Part model, mm, in its own coordinate system. Round coordinates to 2 decimals unless told otherwise and drop trailing zeros. Write each loop counter-clockwise with the first axis right and the second up, starting at its lowest first coordinate (ties: lowest second). Pieces come first, ordered by that corner, then holes. Notation, with made-up numbers: M -24.5,69 L 22.5,69 A30 ccw 22.5,105 Z; hole C 11.5,-20 d7. An arc over 180 degrees is marked long. Use a Markdown table: item, result. Add a question column.
1) Slice it at B-B on z = 0. Write the cut outline in (x, y), plus the area to 4 significant figures.
2) Slice it at D-D on z = -6.5. Write the cut outline in (x, y), plus the area to 3 significant figures.
3) Wall check: probe 1 along X at (y, z) = (2.7, 0); probe 2 along X at (y, z) = (1.6, 0); probe 3 along Z at (x, y) = (-33, 3.25). Give the ranges that are in metal, low to high.
4) Slice it at C-C on x = -58.5. Write the cut outline in (y, z), plus the area to 3 significant figures.
5) Slice it at A-A on y = 3.6. Write the cut outline in (x, z), plus the area to 3 significant figures.
6) Drop flat-ended pins along their axis: P1, Ø1, axis at x = 7, y = 2, coming from the -Z side; P2, Ø3, axis at x = 0, z = 0, coming from the -Y side; P3, Ø1.5, axis at y = 2, z = 1.5, coming from the +X side. Give the stop position or say it passes through.
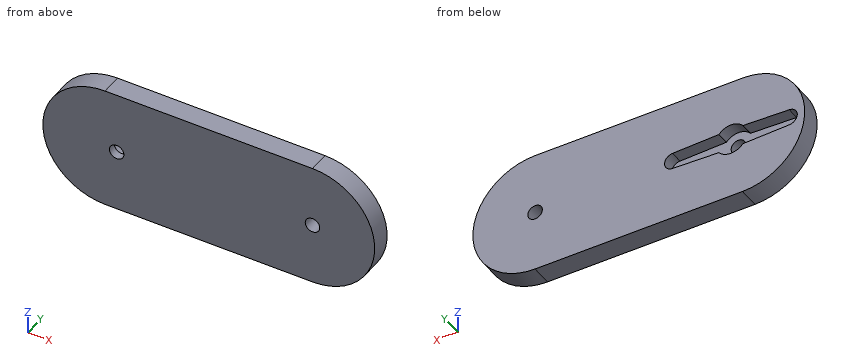
```python
from build123d import *

# Parameters (mm, degrees)
RESSALTO_EXTRUS_O2_DEPTH = 5
ESBO_O4_R                = 1.75
CORTE_EXTRUS_O1_DEPTH    = 10
CORTE_EXTRUS_O2_DEPTH    = 3
ESBO_O7_R                = 2.5
CORTE_EXTRUS_O3_DEPTH    = 3
ESBO_O12_R               = 1.75
CORTE_EXTRUS_O5_DEPTH    = 10


with BuildPart() as part:
    # Esboço3 → Ressalto-extrusão2 (new body)
    with BuildSketch(Plane(origin=(0, 0, 0), x_dir=(1, 0, 0), z_dir=(0, 1, 0))):
        with BuildLine():
            Line((-50, 15), (0, 15))
            ThreePointArc((0, 15), (15, 0), (0, -15))
            Line((0, -15), (-50, -15))
            ThreePointArc((-50, -15), (-65, 0), (-50, 15))
        make_face()
    extrude(amount=RESSALTO_EXTRUS_O2_DEPTH)

    # Esboço4 → Corte-extrusão1 (cut)
    with BuildSketch(Plane(origin=(0, 5, 0), x_dir=(1, 0, 0), z_dir=(0, 1, 0))):
        with Locations(Location((0, 0, 0), (0, 0, 90))):
            Circle(ESBO_O4_R)
    extrude(amount=-CORTE_EXTRUS_O1_DEPTH, mode=Mode.SUBTRACT)

    # Esboço6 → Corte-extrusão2 (cut)
    with BuildSketch(Plane(origin=(0, 5, 0), x_dir=(1, 0, 0), z_dir=(0, 1, 0))):
        with BuildLine():
            Line((-50.096108497, 2.395111434), (-61.281465627, 1.998745461))
            ThreePointArc((-61.281465627, 1.998745461), (-63.210637787, 0), (-61.281465627, -1.998745461))
            Line((-61.281465627, -1.998745461), (-50.096108497, -2.395111434))
            ThreePointArc((-50.096108497, -2.395111434), (-47.210637787, -3.75), (-44.325167077, -2.395111434))
            Line((-44.325167077, -2.395111434), (-33.139809947, -1.998745461))
            ThreePointArc((-33.139809947, -1.998745461), (-31.210637787, 0), (-33.139809947, 1.998745461))
            Line((-33.139809947, 1.998745461), (-44.325167077, 2.395111434))
            ThreePointArc((-44.325167077, 2.395111434), (-47.210637787, 3.75), (-50.096108497, 2.395111434))
        make_face()
        with BuildLine():
            ThreePointArc((-47.443873787, 2.489096416), (-47.210637787, 2.5), (-46.977401787, 2.489096416))
            ThreePointArc((-46.977401787, 2.489096416), (-45.362247947, 1.683286963), (-44.710637787, 0))
            ThreePointArc((-44.710637787, 0), (-45.362247947, -1.683286963), (-46.977401787, -2.489096416))
            ThreePointArc((-46.977401787, -2.489096416), (-47.210637787, -2.5), (-47.443873787, -2.489096416))
            ThreePointArc((-47.443873787, -2.489096416), (-49.710637787, 0), (-47.443873787, 2.489096416))
        make_face(mode=Mode.SUBTRACT)
    extrude(amount=-CORTE_EXTRUS_O2_DEPTH, mode=Mode.SUBTRACT)

    # Esboço7 → Corte-extrusão3 (cut)
    with BuildSketch(Plane(origin=(0, 5, 0), x_dir=(1, 0, 0), z_dir=(0, 1, 0))):
        with Locations((-47.210637787, 0)):
            Circle(ESBO_O7_R)
    extrude(amount=-CORTE_EXTRUS_O3_DEPTH, mode=Mode.SUBTRACT)

    # Esboço12 → Corte-extrusão5 (cut)
    with BuildSketch(Plane(origin=(0, 2, 0), x_dir=(1, 0, 0), z_dir=(0, 1, 0))):
        with Locations(Location((-47.210637787, 0, 0), (0, 0, 270))):
            Circle(ESBO_O12_R)
    extrude(amount=-CORTE_EXTRUS_O5_DEPTH, mode=Mode.SUBTRACT)


solid = part.part
```
Entries:
| question | item | result |
|---|---|---|
| 1 | outline | M -65,0 L -48.96,0 L -48.96,2 L -63.21,2 L -63.21,5 L -65,5 Z; M -45.46,0 L -1.75,0 L -1.75,5 L -31.21,5 L -31.21,2 L -45.46,2 Z; M 1.75,0 L 15,0 L 15,5 L 1.75,5 Z |
| 1 | area | 279.5 mm^2 |
| 2 | outline | M -63.52,0 L 13.52,0 L 13.52,5 L -63.52,5 Z |
| 2 | area | 385 mm^2 |
| 3 | probe 1 | x = -65 to -63.21, -31.21 to -1.75, 1.75 to 15 |
| 3 | probe 2 | x = -65 to -48.96, -45.46 to -1.75, 1.75 to 15 |
| 3 | probe 3 | z = -15 to -1.99, 1.99 to 15 |
| 4 | outline | M 0,-12.36 L 5,-12.36 L 5,-2.1 L 2,-2.1 L 2,2.1 L 5,2.1 L 5,12.36 L 0,12.36 Z |
| 4 | area | 111 mm^2 |
| 5 | outline | M -50,-15 L 0,-15 A15 ccw 0,15 L -50,15 A15 ccw Z; hole M -61.28,-2 L -50.1,-2.4 A3.75 ccw -44.33,-2.4 L -33.14,-2 A2 ccw -33.14,2 L -44.33,2.4 A3.75 ccw -50.1,2.4 L -61.28,2 A2 ccw Z; hole C 0,0 d3.5 |
| 5 | area | 2,050 mm^2 |
| 6 | P1 | stops at z = -13.52 |
| 6 | P2 | passes through |
| 6 | P3 | stops at x = 14.98 |
